```python
from build123d import *

# Parameters (mm, degrees)
F4_DEPTH = 2.8
F5_SIZE  = 1


with BuildPart() as f1:
    # F0 (on Front) → F1 (revolve)
    with BuildSketch(Plane.XZ):
        Polygon((0, 35.5), (0, 0), (77, 0), (77, 9), (54, 9), (54, 12), (24, 12), (24, 35.5), (16.924277, 35.5), (14, 26.5), (10, 26.5), (7.075723, 35.5), align=None)
    revolve(axis=Axis((38.5, 0, 0), (1, 0, 0)))

    # F3 (on offset) → F4 (cut)
    with BuildSketch(Plane.XY.offset(9)):
        with BuildLine():
            Line((57, -3), (77, -3))
            Line((77, -3), (77, 3))
            Line((77, 3), (57, 3))
            ThreePointArc((57, 3), (54, 0), (57, -3))
        make_face()
    extrude(amount=-F4_DEPTH, mode=Mode.SUBTRACT)

    # F5
    f5_edges = [f1.edges().sort_by_distance(p)[0] for p in [
        (77, 0, -9),
    ]]
    chamfer(f5_edges, length=F5_SIZE)


solid = f1.part
```
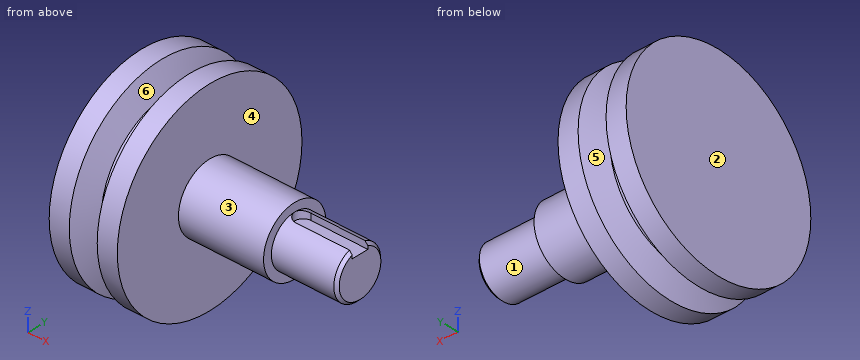
Geometry: final body of the model. Coordinates: model frame, mm. Face numbers are marked on the shaded views. A direction names the side the tool comes from. Coordinates: 2 decimals unless noted, no trailing zeros. Order: outer loops, then holes, each group sorted by start corner. A loop starts at its lowest first (then second) coordinate and runs counter-clockwise, first axis right, second up. Notation, with made-up numbers: M 41.5,-31.75 L 65.5,-31.75 A30 cw 65.5,6.25 Z; hole C -4.75,-7 d6. An arc over 180 degrees is marked long. Answer as CSV lines item,"result".
Q1. Section B-B on x = 70. Return the cut outline in (y, z), and give its area (3 significant figures).
Answers:
outline,"M -3,6.2 L -3,8.49 A9 ccw long 3,8.49 L 3,6.2 Z"
area,"239 mm^2"
Q2. Section A-A on z = 0. Return the cut outline in (x, y), and give its area (3 significant figures).
Answers:
outline,"M 0,-35.5 L 7.08,-35.5 L 10,-26.5 L 14,-26.5 L 16.92,-35.5 L 24,-35.5 L 24,-12 L 54,-12 L 54,-9 L 76,-9 L 77,-8 L 77,8 L 76,9 L 54,9 L 54,12 L 24,12 L 24,35.5 L 16.92,35.5 L 14,26.5 L 10,26.5 L 7.08,35.5 L 0,35.5 Z"
area,"2,710 mm^2"
Q3. Draft query along X for the marked faces 3, 4, 5 and 6. Return one class per face: pulls with the +X half, pulls with the -X half, needs draft (parallel to the pull), parting line crosses it, or undercut.
Answers:
face 3,"needs draft"
face 4,"pulls with the +X half"
face 5,"undercut"
face 6,"undercut"
Q4. Line query: probe 1 along X at (y, z) = (-9.5, 5.5); probe 2 along X at (y, z) = (-20, 9); probe 3 along X at (y, z) = (8, -31). Output: solid intervals per line, ascending. Write a range as [from, to].
Answers:
probe 1,"x = [0, 54]"
probe 2,"x = [0, 24]"
probe 3,"x = [0, 8.21], [15.79, 24]"
Q5. Section C-C on x = 52. Return the cut outline in (y, z), and give its area (3 significant figures).
Answers:
outline,"C 0,0 d24"
area,"452 mm^2"
Q6. Set-up query: the marked faces 1 and 2. Return all of +Z, -Z, +X, -X, +Y, -Y with unobstructed straight access to the full face (end or side cutting, diameter ignored); none if empty.
Answers:
face 1,"+X"
face 2,"+Z, -Z, -X, +Y, -Y"
Q7. First-contact query: P1, Ø6.5, axis at x = 66, y = 1, coming from the +Z side; P2, Ø2.5, axis at x = 64.5, z = 7.5, coming from the -Y side; P3, Ø6, axis at x = 37, y = 0.5, coming from the +Z side. Flat tips, straight axial feed; report the tip coordinate or a pass-through.
Answers:
P1,"stops at z = 8.49"
P2,"stops at y = -6.48"
P3,"stops at z = 12"
